Check sheet for the modelled part. Datum: model origin and axes. Units: mm. Face numbers are marked on the shaded views. Coordinates: 2 decimals unless noted, no trailing zeros. Write each loop counter-clockwise with the first axis right and the second up, starting at its lowest first coordinate (ties: lowest second). Pieces come first, ordered by that corner, then holes. Notation, with made-up numbers: (76, -19) -> (90, -19) arc R29 ccw to (90, 18) -> close; hole circle Ø2 at (-32.75, 56.5). An arc over 180 degrees is marked (long way). One line per item, written item: value. Start each with the question number.
1) Scan lines: line 1 along X through (y, z) = (1, -4.5); line 2 along Z through (x, y) = (-9.5, 0); line 3 along Y through (x, z) = (-11.5, -6.5). Record each from-to range of solid material in increasing order. Write a range as [from, to].
2) Sectioned sample at C-C on x = -3. Enter the section's corners in (y, z).
3) Draft check along X on the marked faces 1 and 2. Enter one of: +X half, -X half, draft (parallel to the pull), parting line (faces both ways), or undercut.
4) Sectioned sample at A-A on z = -4.5. Enter the section's corners in (x, y), plus the area to 3 significant figures.
5) Sectioned sample at B-B on y = 15. Enter the section's corners in (x, z), plus the area to 3 significant figures.
6) Gauge pin test, flat ends, axial feed: P1, Ø1.5, axis at x = 12.5, y = 9, coming from the -Z side; P2, Ø4, axis at y = 28.5, z = -17, coming from the -X side; P3, Ø12, axis at x = 8.5, y = 14, coming from the +Z side; P4, Ø12, axis at x = -11, y = 7.5, coming from the -Z side. Record the tip position at first contact, or that the pin passes through.
Autodesk Inventor part; units mm, degrees
ref_plane "Work Plane7" through (-5.4512, 35.4213, -181.4907) normal (0.0029789, 0.9999956, 0) x (0, 0, 1)
ref_plane "Work Plane8" through (-5.4751, 27.4214, -181.4903) normal (-0.0029789, -0.9999956, 0) x (0.9999956, -0.0029789, 0)
ref_plane "YZ Plane" through (0, 0, 0) normal (1, 0, 0) x (0, 1, 0)
ref_plane "Work Plane5" through (16.1538, -3.6432, -7.1) normal (0.0029789, 0.9999956, 0) x (0, 0, 1)
sketch "Sketch5" plane through (16.1538, -3.6432, -7.1) normal (0.0029789, 0.9999956, 0) x (0, 0, 1)
  circle A0 centre (-16.4, -26.2) radius 1.75
  circle A1 centre (-16.4, -6.2) radius 1.75
  line L0 (0, -32.4) -> (6.5, -32.4)
  line L1 (6.5, 0) -> (6.5, -32.4)
  line L2 (0, 0) -> (6.5, 0)
  line L3 (0, 0) -> (0, -32.4)
  circle A2 centre (3.6, -6.2) radius 1.75
  circle A3 centre (3.6, -26.2) radius 1.75
  line L4 (-19.9, 0) -> (-19.9, -32.4)
  line L5 (6.5, -32.4) -> (-19.9, -32.4)
  line L6 (-19.9, -32.4) -> (-19.9, 0)
  line L7 (-19.9, 0) -> (6.5, 0)
  line L8 (6.5, 0) -> (6.5, -32.4)
  point P0 (7.1, -16.1645)
extrude "Extrusion4" add sketch "Sketch5" along normal blind 8
sketch "Sketch7" plane through (16.1776, 4.3568, -7.1) normal (0.0029789, 0.9999956, 0) x (0.9999956, -0.0029789, 0)
  point P0 (-16.1645, -7.1)
sketch "Sketch8" plane through (16.1776, 4.3568, -7.1) normal (0.0029789, 0.9999956, 0) x (0.9999956, -0.0029789, 0)
  circle A0 centre (-26.2, -3.6) radius 1.75
  circle A1 centre (-6.2, -3.6) radius 1.75
  circle A2 centre (-6.2, 16.4) radius 1.75
  circle A3 centre (-26.2, 16.4) radius 1.75
  line L0 (-32.4, -6.5) -> (0, -6.5)
  line L1 (0, -6.5) -> (0, 19.9)
  line L2 (0, 19.9) -> (-32.4, 19.9)
  line L3 (-32.4, 19.9) -> (-32.4, -6.5)
  circle A4 centre (-16.2177, 39.3896) radius 1.75
  line L4 (-22.2006, -0.6104) -> (-22.0458, -0.6104)
  line L5 (-22.2, -0.6104) -> (-22.2, -0.6104)
  line L6 (-22.2, -0.6104) -> (-21.7015, -0.6104)
  line L7 (-21.7015, -0.6104) -> (-14.6224, -0.6104)
  line L8 (-14.6224, -0.6104) -> (-13.8248, -0.6104)
  line L9 (-13.8248, -0.6104) -> (-10.7339, -0.6104)
  line L10 (-10.7339, -0.6104) -> (-10.2354, -0.6104)
  line L11 (-10.2354, -0.6104) -> (-10.2354, -0.6104)
  line L12 (-10.3901, -0.6104) -> (-10.2354, -0.6104)
  line L13 (-10.966, -0.6104) -> (-10.3901, -0.6104)
  line L14 (-11.1588, -0.6104) -> (-10.966, -0.6104)
  line L15 (-11.1588, -0.6104) -> (-11.5034, -0.6104)
  line L16 (-11.731, -0.6104) -> (-11.5034, -0.6104)
  line L17 (-11.731, -0.6104) -> (-11.731, -0.6104)
  line L18 (-11.731, -0.6104) -> (-11.5034, -0.6104)
  line L19 (-11.5034, -0.6104) -> (-11.1379, -0.6104)
  line L20 (-11.1379, -0.6104) -> (-10.9487, -0.6104)
  line L21 (-10.9487, -0.6104) -> (-10.3901, -0.6104)
  line L22 (-10.3901, -0.6104) -> (-10.2354, -0.6104)
  line L23 (-10.2354, -0.6104) -> (-10.2354, -0.6104)
  line L24 (-10.2354, -0.6104) -> (-10.7339, -0.6104)
  line L25 (-10.7339, -0.6104) -> (-21.7015, -0.6104)
  line L26 (-21.7015, -0.6104) -> (-22.2, -0.6104)
  line L27 (-22.2, -0.6104) -> (-22.2, -0.6104)
  line L28 (-22.2001, -0.6104) -> (-22.0454, -0.6104)
  line L29 (-22.0454, -0.6104) -> (-21.4867, -0.6104)
  line L30 (-21.4867, -0.6104) -> (-21.2975, -0.6104)
  line L31 (-21.2975, -0.6104) -> (-20.932, -0.6104)
  line L32 (-20.932, -0.6104) -> (-20.7045, -0.6104)
  line L33 (-20.7045, -0.6104) -> (-20.7045, -0.6104)
  line L34 (-20.932, -0.6104) -> (-20.7045, -0.6104)
  line L35 (-20.932, -0.6104) -> (-21.2766, -0.6104)
  line L36 (-21.4694, -0.6104) -> (-21.2766, -0.6104)
  line L37 (-22.0458, -0.6104) -> (-21.4694, -0.6104)
  line L38 (-32.4, 19.9) -> (-32.4, -6.5)
  line L39 (-32.4, 5.9) -> (-21.4, 16.9)
  line L40 (-21.4, 16.9) -> (-11, 16.9)
  line L41 (-11, 16.9) -> (0, 5.9)
  line L42 (0, -6.5) -> (0, 19.9)
  line L43 (0, 1.5) -> (-32.4, 1.5)
  line L44 (-32.4, 5.9) -> (-32.4, -0.0368)
  line L45 (0, 5.9) -> (0, 1.5)
  circle A5 centre (-16.2177, 9.3896) radius 1.75
  circle A6 centre (-16.2177, 9.3896) radius 1.4
  point P0 (-16.1645, -7.1)
  dimension "d25" = 45
  dimension "d26" = 45
  dimension "d27" = 3
  dimension "d28" = 11
  dimension "d29" = 11
  dimension "d30" = 8
  dimension "d46" = 2.8
ref_plane "Work Plane7" through (-5.4512, 35.4213, -181.4907) normal (0.0029789, 0.9999956, 0) x (0, 0, 1)
extrude "Extrusion5" add sketch "Sketch8" along normal up to surface (31 mm away) contours L43 L3 L39 L40 L41 L1 | A5
sketch "Sketch9" plane through (16.2699, 35.3566, -8.6) normal (0.0029789, 0.9999956, 0) x (0.9999956, -0.0029789, 0)
  line L0 (-22.2, -2.1104) -> (-22.2, 197.8896)
  line L1 (-10.2354, -2.1104) -> (-10.2354, 197.8896)
  line L2 (-22.5, 20.2984) -> (-9.9354, 20.2984)
  line L3 (-9.9354, 20.2984) -> (-9.9354, -1.0464)
  line L4 (-9.9354, -1.0464) -> (-22.5, -1.0464)
  line L5 (-22.5, -1.0464) -> (-22.5, 20.2984)
  point P0 (-16.1645, -8.6)
  dimension "d34" = 0.3
  dimension "d35" = 0.3
ref_plane "Work Plane8" through (-5.4751, 27.4214, -181.4903) normal (-0.0029789, -0.9999956, 0) x (0.9999956, -0.0029789, 0)
extrude "Extrusion6" cut sketch "Sketch9" against normal up to surface (8 mm away)
sketch "Sketch10" plane through (-16.2461, -3.5467, -27) normal (-0.9999956, 0.0029789, 0) x (0, 0, 1)
  line L0 (0, 0) -> (26.4, 0)
  line L1 (26.4, 0) -> (26.4, 8)
  line L2 (18.4, 8) -> (26.4, 8)
  line L3 (0, 0) -> (0, 8)
  circle A0 centre (14.8051, 35.8681) radius 1.4
  line L4 (18.4, 8) -> (18.4, 39)
  line L5 (18.4, 39) -> (14, 39)
  line L6 (14, 8) -> (14, 39)
  line L7 (0, 8) -> (14, 8)
  point P0 (27, 3.595)
  dimension "d38" = 2.8
extrude "Extrusion7" cut sketch "Sketch10" against normal through all contours L6 A0 | A0 L6
sketch "Sketch11" plane through (-16.2223, 4.4533, -8.6) normal (0, 0, 1) x (0.9999956, -0.0029789, 0)
  circle A0 centre (16.2, 7.5) radius 5.65
  circle A1 centre (16.2, 7.5) radius 6.35
  point P0 (16.2355, -4.405)
  dimension "d41" = 0.7
extrude "Extrusion8" cut sketch "Sketch11" against normal through all contours A0 | A1
sketch "Sketch12" plane through (-16.2223, 4.4533, -8.6) normal (0, 0, 1) x (0.9999956, -0.0029789, 0)
  line L0 (3.2, 25.4) -> (-3.8, 25.4)
  line L1 (3.2, 25.4) -> (3.2, 69.4)
  line L2 (-3.8, 69.4) -> (3.2, 69.4)
  line L3 (3.2, 18.4) -> (3.2, 26.4)
  line L4 (-2.7347, 16.1972) -> (5.1158, 16.1972)
  line L5 (5.1158, 16.1972) -> (5.1158, 65.2014)
  line L6 (5.1158, 65.2014) -> (-2.7347, 65.2014)
  line L7 (-2.7347, 65.2014) -> (-2.7347, 16.1972)
  line L8 (-3.8, 25.4) -> (-3.8, 69.4)
  line L9 (-3.8, 18.4) -> (3.2, 18.4)
  line L10 (-3.8, 26.4) -> (-3.8, 18.4)
  line L11 (3.2, 26.4) -> (-3.8, 26.4)
  point P0 (16.2355, -4.405)
  point P1 (-1.8, 18.4)
  point P2 (-1.8, 26.4)
extrude "Extrusion9" cut sketch "Sketch12" against normal through all contours L3 L9 L7 L0 | L0 L7 L11 L1 | L1 L6 L5 L4 L7 L9 L3 | L11 L7 L6 L1
properties part number "03_Support_Xslide"
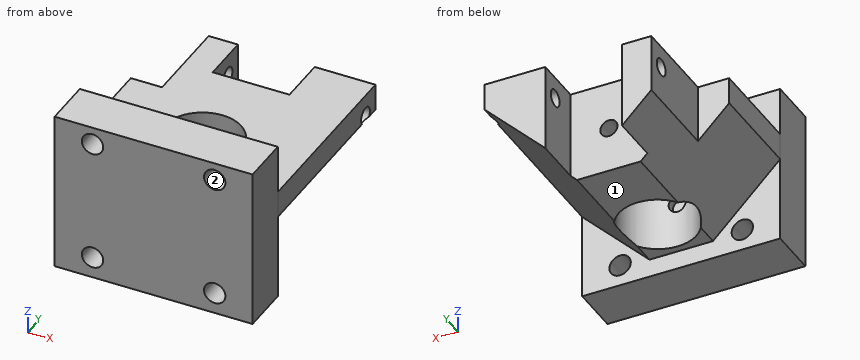
Answers:
1. line 1: x = [-16.23, -11.47], [-8.6, 8.53], [11.4, 16.17]
1. line 2: z = [-27, -25.17], [-21.83, -5.17], [-1.83, -0.6]
1. line 3: y = [-3.56, 4.44]
2. outline: (-3.59, -27) -> (4.41, -27) -> (4.41, -24) -> (6.31, -24) -> (6.31, -8.6) -> (4.41, -8.6) -> (4.41, -0.6) -> (-3.59, -0.6) -> close; (17.5, -24) -> (27.41, -24) -> (27.41, -8.6) -> (17.5, -8.6) -> close
3. face 1: draft
3. face 2: undercut
4. outline: (-16.25, -3.55) -> (-11.48, -3.56) -> (-11.46, 4.44) -> (-16.22, 4.45) -> close; (-8.61, -3.57) -> (8.52, -3.62) -> (8.54, 4.38) -> (-8.59, 4.43) -> close; (11.39, -3.63) -> (16.15, -3.64) -> (16.18, 4.36) -> (11.41, 4.37) -> close
4. area: 213 mm2
5. outline: (-16.19, -13) -> (-5.54, -23.65) -> (-5.54, -8.6) -> (-16.19, -8.6) -> close; (5.54, -23.66) -> (16.21, -13) -> (16.21, -8.6) -> (5.54, -8.6) -> close
5. area: 207 mm2
6. P1: stops at z = -17.44
6. P2: stops at x = -11.04
6. P3: stops at z = -8.6
6. P4: stops at z = -27
